Can you work these out from the model? Positions are in its coordinate system, mm. Coordinates: 2 decimals unless noted, no trailing zeros. Order: outer loops, then holes, each group sorted by start corner. A loop starts at its lowest first (then second) coordinate and runs counter-clockwise, first axis right, second up. Notation, with made-up numbers: (54, 4) -> (106, 4) arc R7 cw to (106, 17) -> close; hole circle Ø6 at (80.5, -13.75). An arc over 180 degrees is marked (long way). Answer as CSV lines item,"result".
from build123d import *

# Parameters (mm, degrees)
F0_R     = 1.6
F1_DEPTH = 3.175


# Not quite as in the source:
# - a length typed as a fraction of an inch, garbled in the dataset ("3 / 203.2 mm" for 3/8 in), is restored


with BuildPart() as f1:
    # F0 (on Front) → F1 (new body)
    with BuildSketch(Plane.XZ):
        with BuildLine():
            Line((37.46, 0), (2.54, 0))
            ThreePointArc((2.54, 0), (0.7439487758, -0.7439487758), (0, -2.54))
            Line((0, -2.54), (0, -37.46))
            ThreePointArc((0, -37.46), (0.7439487758, -39.2560512242), (2.54, -40))
            Line((2.54, -40), (37.46, -40))
            ThreePointArc((37.46, -40), (39.2560512242, -39.2560512242), (40, -37.46))
            Line((40, -37.46), (40, -2.54))
            ThreePointArc((40, -2.54), (39.2560512242, -0.7439487758), (37.46, 0))
        make_face()
        with Locations((5, -35)):
            Circle(F0_R, mode=Mode.SUBTRACT)
        with Locations((15, -35)):
            Circle(F0_R, mode=Mode.SUBTRACT)
        with Locations((5, -25)):
            Circle(F0_R, mode=Mode.SUBTRACT)
        with Locations((15, -25)):
            Circle(F0_R, mode=Mode.SUBTRACT)
        with Locations((25, -35)):
            Circle(F0_R, mode=Mode.SUBTRACT)
        with Locations((35, -35)):
            Circle(F0_R, mode=Mode.SUBTRACT)
        with Locations((25, -25)):
            Circle(F0_R, mode=Mode.SUBTRACT)
        with Locations((35, -25)):
            Circle(F0_R, mode=Mode.SUBTRACT)
        with Locations((5, -15)):
            Circle(F0_R, mode=Mode.SUBTRACT)
        with Locations((15, -15)):
            Circle(F0_R, mode=Mode.SUBTRACT)
        with Locations((5, -5)):
            Circle(F0_R, mode=Mode.SUBTRACT)
        with Locations((15, -5)):
            Circle(F0_R, mode=Mode.SUBTRACT)
        with Locations((25, -15)):
            Circle(F0_R, mode=Mode.SUBTRACT)
        with Locations((35, -15)):
            Circle(F0_R, mode=Mode.SUBTRACT)
        with Locations((25, -5)):
            Circle(F0_R, mode=Mode.SUBTRACT)
        with Locations((35, -5)):
            Circle(F0_R, mode=Mode.SUBTRACT)
    extrude(amount=F1_DEPTH)


solid = f1.part
Q1. Imagine slicing it at A-A (z = -15). List the corners of the cut face in (x, y) for me (3 decimals), and give its area (3 significant figures).
Solution:
outline,"(0, -3.175) -> (3.4, -3.175) -> (3.4, 0) -> (0, 0) -> close; (6.6, -3.175) -> (13.4, -3.175) -> (13.4, 0) -> (6.6, 0) -> close; (16.6, -3.175) -> (23.4, -3.175) -> (23.4, 0) -> (16.6, 0) -> close; (26.6, -3.175) -> (33.4, -3.175) -> (33.4, 0) -> (26.6, 0) -> close; (36.6, -3.175) -> (40, -3.175) -> (40, 0) -> (36.6, 0) -> close"
area,"86.4 mm2"
Q2. If I drill on line 1 (Z direction, x = 35, y = -0.3); line 2 (X direction, y = -0.25, z = -24); line 3 (Z direction, x = 25.5, y = -1.35), over which ranges is the centre line in solid material (lowest first)?
Solution:
line 1,"-40 to -36.6, -33.4 to -26.6, -23.4 to -16.6, -13.4 to -6.6, -3.4 to 0"
line 2,"0 to 3.75, 6.25 to 13.75, 16.25 to 23.75, 26.25 to 33.75, 36.25 to 40"
line 3,"-40 to -36.52, -33.48 to -26.52, -23.48 to -16.52, -13.48 to -6.52, -3.48 to 0"
Q3. We'd pull the mould along Z, two halves only. Please class faces 1 (the flat face through (20, 0, -20)), 2 (the cylindrical face through (33.82, -1.57, -13.92)), 3 (the cylindrical face through (0.764, -1.565, -0.724)): pulls with the +Z half, pulls with the -Z half, needs draft (parallel to the pull), parting line crosses it, or undercut.
Solution:
face 1,"needs draft"
face 2,"undercut"
face 3,"pulls with the +Z half"
Q4. Imagine slicing it at B-B (y = -1.8). Give the number of separate pieces and of enclosed holes in the cut face, and give its area (3 significant figures).
Solution:
separate pieces,"1"
enclosed holes,"16"
area,"1,470 mm2"
Q5. Imagine slicing it at C-C (x = 15). List the corners of the cut face in (y, z) for me (3 decimals).
Solution:
outline,"(-3.175, -40) -> (0, -40) -> (0, -36.6) -> (-3.175, -36.6) -> close; (-3.175, -33.4) -> (0, -33.4) -> (0, -26.6) -> (-3.175, -26.6) -> close; (-3.175, -23.4) -> (0, -23.4) -> (0, -16.6) -> (-3.175, -16.6) -> close; (-3.175, -13.4) -> (0, -13.4) -> (0, -6.6) -> (-3.175, -6.6) -> close; (-3.175, -3.4) -> (0, -3.4) -> (0, 0) -> (-3.175, 0) -> close"
